Build history of the part. All positions in model axes, mm. Coordinates: 2 decimals unless noted, no trailing zeros. Order: outer loops, then holes, each group sorted by start corner. A loop starts at its lowest first (then second) coordinate and runs counter-clockwise, first axis right, second up. Notation, with made-up numbers: (51, 6) -> (76, 6) arc R29 ccw to (76, 31) -> close; hole circle Ø2 at (-6, 50.25). An arc over 180 degrees is marked (long way). Write each question's results on one line, items separated by ' | '.
Solid Edge part; units mm, degrees
sketch "Sketch1" plane through (0, 0, 0) normal (0, 0, 1) x (1, 0, 0)
  circle A0 centre (0, 0) radius 37
  circle A1 centre (0, 0) radius 27.8
extrude "Protrusion1" add sketch "Sketch1" along normal blind 2
sketch "Sketch2" plane through (0, 0, 2) normal (0, 0, 1) x (1, 0, 0)
  circle A0 centre (-32.5, 0) radius 3.15
  circle A1 centre (-31.5556, 7.7778) radius 3.15
  circle A2 centre (-28.7773, 15.1035) radius 3.15
  circle A3 centre (-24.3266, 21.5515) radius 3.15
  circle A4 centre (-18.4621, 26.747) radius 3.15
  circle A5 centre (-11.5247, 30.388) radius 3.15
  circle A6 centre (-3.9174, 32.263) radius 3.15
  circle A7 centre (3.9174, 32.263) radius 3.15
  circle A8 centre (11.5247, 30.388) radius 3.15
  circle A9 centre (18.4621, 26.747) radius 3.15
  circle A10 centre (24.3266, 21.5515) radius 3.15
  circle A11 centre (28.7773, 15.1035) radius 3.15
  circle A12 centre (31.5556, 7.7778) radius 3.15
  circle A13 centre (32.5, 0) radius 3.15
  circle A14 centre (31.5556, -7.7778) radius 3.15
  circle A15 centre (28.7773, -15.1035) radius 3.15
  circle A16 centre (24.3266, -21.5515) radius 3.15
  circle A17 centre (18.4621, -26.747) radius 3.15
  circle A18 centre (11.5247, -30.388) radius 3.15
  circle A19 centre (3.9174, -32.263) radius 3.15
  circle A20 centre (-3.9174, -32.263) radius 3.15
  circle A21 centre (-11.5247, -30.388) radius 3.15
  circle A22 centre (-18.4621, -26.747) radius 3.15
  circle A23 centre (-24.3266, -21.5515) radius 3.15
  circle A24 centre (-28.7773, -15.1035) radius 3.15
  circle A25 centre (-31.5556, -7.7778) radius 3.15
extrude "Cutout1" cut sketch "Sketch2" against normal up to next
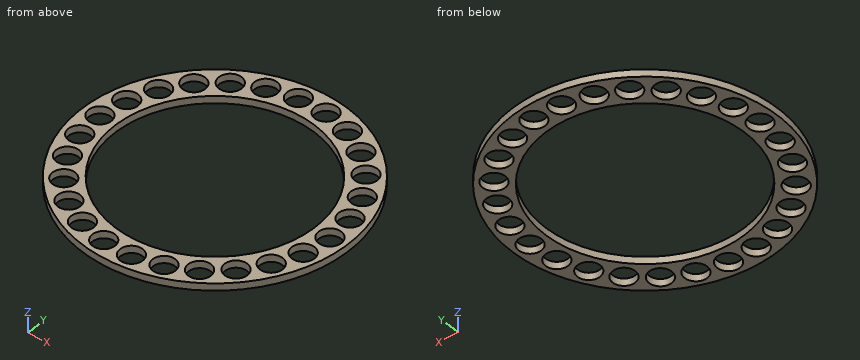
Item 1: Slice it at A-A, the plane x = 5. List the corners of the cut face in (y, z).
Answer:
outline: (-36.66, 0) -> (-35.22, 0) -> (-35.22, 2) -> (-36.66, 2) -> close; (-29.3, 0) -> (-27.35, 0) -> (-27.35, 2) -> (-29.3, 2) -> close; (27.35, 0) -> (29.3, 0) -> (29.3, 2) -> (27.35, 2) -> close; (35.22, 0) -> (36.66, 0) -> (36.66, 2) -> (35.22, 2) -> close
Item 2: Drill centre lines: line 1 (X direction, y = -28, z = 0.9); line 2 (X direction, y = -24, z = 1.5); line 3 (X direction, y = 20, z = 1.55). Where is each one in solid material? Low to high. Write a range as from..to.
Answer:
line 1: x = -24.19..-21.35, -15.57..-13.58, -9.47..9.47, 13.58..15.57, 21.35..24.19 | line 2: x = -28.16..-26.31, -22.34..-20, -16.92..-14.03, 14.03..16.92, 20..22.34, 26.31..28.16 | line 3: x = -31.13..-27.07, -21.59..-19.31, 19.31..21.59, 27.07..31.13
Item 3: Slice it at C-C, the plane z = 0.3. State how many separate pieces and enclosed holes the cut face has, and give its area (3 significant figures).
Answer:
separate pieces: 1 | enclosed holes: 27 | area: 1,060 mm^2
Item 4: Pin check, flat tips, straight feed: pin 1 (5.5 mm diameter, centred on x = 32.5, y = 0, fed in from -Z); pin 2 (1 mm diameter, centred on y = 22.5, z = 1.5, fed in from +X); pin 3 (1 mm diameter, centred on x = 15.5, z = 1, fed in from +Y). Stop position of each tip, or through.
Answer:
pin 1: passes through | pin 2: stops at x = 29.75 | pin 3: stops at y = 33.82
Item 5: Slice it at B-B, the plane y = 13. List the corners of the cut face in (x, z), and give its area (3 significant figures).
Answer:
outline: (-34.64, 0) -> (-31.12, 0) -> (-31.12, 2) -> (-34.64, 2) -> close; (-26.43, 0) -> (-24.57, 0) -> (-24.57, 2) -> (-26.43, 2) -> close; (24.57, 0) -> (26.43, 0) -> (26.43, 2) -> (24.57, 2) -> close; (31.12, 0) -> (34.64, 0) -> (34.64, 2) -> (31.12, 2) -> close | area: 21.5 mm^2
